from build123d import *

# Parameters (mm, degrees)
SKETCH1_R           = 70
BOSS_EXTRUDE1_DEPTH = 25
BOSS_EXTRUDE2_DEPTH = 10
BOSS_EXTRUDE3_START = 0.1
SKETCH27_R          = 70
BOSS_EXTRUDE3_DEPTH = 0.1
SHELL3_START        = -0.1
SHELL3_OUTLINE_R    = 68
SHELL3_DEPTH        = 23.1
SHELL3_START_2      = 2
SHELL3_2_DEPTH      = 6


# Read off the part's stored shape, not the designer's step: Shell3
with BuildPart() as part:
    # Sketch1 → Boss-Extrude1 (new body)
    with BuildSketch(Plane.XY):
        Circle(SKETCH1_R)
    extrude(amount=BOSS_EXTRUDE1_DEPTH)

    # Sketch21 → Boss-Extrude2 (add)
    with BuildSketch(Plane.XY):
        with BuildLine():
            Line((-13.97898065, -68.59), (-6, -85.59))
            ThreePointArc((-6, -85.59), (0, -91.59), (6, -85.59))
            Line((6, -85.59), (13.97898065, -68.59))
            ThreePointArc((13.97898065, -68.59), (0, -70), (-13.97898065, -68.59))
        make_face()
    extrude(amount=BOSS_EXTRUDE2_DEPTH)

    # Sketch27 → Boss-Extrude3 (add)
    with BuildSketch(Plane(origin=(0, 0, 0), x_dir=(-1, 0, 0), z_dir=(0, 0, -1)).offset(BOSS_EXTRUDE3_START)):
        Circle(SKETCH27_R)
    extrude(amount=-BOSS_EXTRUDE3_DEPTH)

    # Shell3 outline → Shell3 (cut)
    with BuildSketch(Plane.XY.offset(SHELL3_START)):
        Circle(SHELL3_OUTLINE_R)
    extrude(amount=SHELL3_DEPTH, mode=Mode.SUBTRACT)

    # Shell3 2 outline → Shell3 2 (cut)
    with BuildSketch(Plane.XY.offset(SHELL3_START_2)):
        with BuildLine():
            ThreePointArc((12.599173957, -66.82260707), (0, -68), (-12.599173957, -66.82260707))
            Line((-12.599173957, -66.82260707), (-3.979676533, -85.187290811))
            ThreePointArc((-3.979676533, -85.187290811), (0, -89.59), (3.979676533, -85.187290811))
            Line((3.979676533, -85.187290811), (12.599173957, -66.82260707))
        make_face()
    extrude(amount=SHELL3_2_DEPTH, mode=Mode.SUBTRACT)


solid = part.part
Geometry check sheet. Reference: the model listing, model coordinates, mm. A direction names the side the tool comes from. Give positions to 0.01 mm unless a question says otherwise; leave off trailing zeros. Loops run counter-clockwise (first coordinate to the right, second up) from the corner with the lowest first, then second, coordinate; pieces in that order, holes last. Notation, with made-up numbers: M 5.5,5.25 L 38.5,5.25 A26 ccw 38.5,34.25 Z; hole C 49,-15 d5. An arc over 180 degrees is marked long. Answer as a JSON object with one key per item and string values. Group by question number.
Item 1: Mould release check, pull along Z, two halves, no side actions. Record for faces 1 (the flat face through (-1, 1, 25)), 2 (the flat face through (11, 68, -0.1)), 3 (the flat face through (0, -76, 8)): pulls with the +Z half, pulls with the -Z half, needs draft (parallel to the pull), parting line crosses it, or undercut.
Item 2: Sectioned sample at C-C on x = 0. Record the boundary of the cut face in (y, z), plus the area to 3 significant figures.
Item 3: Sectioned sample at B-B on y = 0. Record the boundary of the cut face in (x, z), plus the area to 3 significant figures.
Item 4: Gauge pin test, flat ends, axial feed: pin 1 (1.5 mm diameter, centred on y = -46.5, z = 5.5, fed in from -X); pin 2 (4 mm diameter, centred on x = 23.5, z = 10, fed in from +Y); pin 3 (13 mm diameter, centred on x = 0, y = -85.59, fed in from -Z). Record the tip position at first contact, or that the pin passes through.
Item 5: Sectioned sample at A-A on z = 4.5. Record the boundary of the cut face in (x, y), plus the area to 3 significant figures.
Item 6: Material ranges on L1, parallel to X at y = -85.59, z = 5.25; L2, parallel to X at y = 1.5, z = 8.5; L3, parallel to Y at x = 0, z = 5.85, recorded low to high.
Item 7: Access from +Z, -Z, +X, -X, +Y, -Y to the whole of each face (thin tool, end or side, straight path). Record for faces 4 (the cylindrical face through (36.556, 57.338, 11.288)), 5 (the flat face through (-10.045, -76.971, 4.93)), 6 (the flat face through (8.23, -76.13, 4.96)).
Item 8: Sectioned sample at D-D on y = -77. Record the boundary of the cut face in (x, z).
Findings below:
{
 "1": {"face 1": "pulls with the +Z half", "face 2": "pulls with the -Z half", "face 3": "undercut"},
 "2": {"outline": "M -91.59,0 L -70,0 L -70,-0.1 L -68,-0.1 L -68,2 L -89.59,2 L -89.59,8 L -68,8 L -68,23 L 68,23 L 68,-0.1 L 70,-0.1 L 70,25 L -70,25 L -70,10 L -91.59,10 Z", "area": "459 mm2"},
 "3": {"outline": "M -70,-0.1 L -68,-0.1 L -68,23 L 68,23 L 68,-0.1 L 70,-0.1 L 70,25 L -70,25 Z", "area": "372 mm2"},
 "4": {"pin 1": "x = -52.98", "pin 2": "y = 66.62", "pin 3": "z = 0"},
 "5": {"outline": "M -13.98,-68.59 L -6,-85.59 A6 ccw 6,-85.59 L 13.98,-68.59 A70 ccw long Z; hole M -12.6,-66.82 L -3.98,-85.19 A4 ccw long 3.98,-85.19 L 12.6,-66.82 A68 ccw long Z", "area": "924 mm2"},
 "6": {"L1": "-6 to -4, 4 to 6", "L2": "-69.98 to -67.98, 67.98 to 69.98", "L3": "-91.59 to -89.59, 68 to 70"},
 "7": {"face 4": "-Z", "face 5": "+Z, -Z, -X, -Y", "face 6": "none"},
 "8": {"outline": "M -10.03,0 L 10.03,0 L 10.03,10 L -10.03,10 Z; hole M -7.82,2 L 7.82,2 L 7.82,8 L -7.82,8 Z"}
}
